from build123d import *

# Parameters (mm, degrees)
F0_R     = 38.1
F0_R_2   = 19.05
F1_DEPTH = 76.2
F2_R     = 9.52499
F4_R     = 31.75
F4_R_2   = 25.4
F5_DEPTH = 3.175
F6_R     = 3.17499
F8_R     = 19.05
F9_DEPTH = 152.4


# Not quite as in the source:
# - a fillet or chamfer is up to 0.001 mm smaller than in the source, because OpenCascade refuses the exact size


with BuildPart() as f1:
    # F0 (on Front) → F1 (new body, symmetric)
    with BuildSketch(Plane.XZ):
        Circle(F0_R)
        Circle(F0_R_2, mode=Mode.SUBTRACT)
    extrude(amount=F1_DEPTH, both=True)

    # F2 (radius 9.525 in the source; OpenCascade refuses exactly that, so slightly less here)
    f2_edges = [f1.edges().sort_by_distance(p)[0] for p in [
        (-38.1, -76.2, 0),
        (-19.05, -76.2, 0),
    ]]
    fillet(f2_edges, radius=F2_R)

    # F4 (on offset) → F5 (cut)
    with BuildSketch(Plane(origin=(0, 76.2, 0), x_dir=(-1, 0, 0), z_dir=(0, 1, 0))):
        Circle(F4_R)
        Circle(F4_R_2, mode=Mode.SUBTRACT)
    extrude(amount=-F5_DEPTH, mode=Mode.SUBTRACT)

    # F6 (radius 3.175 in the source; OpenCascade refuses exactly that, so slightly less here)
    f6_edges = [f1.edges().sort_by_distance(p)[0] for p in [
        (31.75, 73.025, 0),
        (25.4, 73.025, 0),
    ]]
    fillet(f6_edges, radius=F6_R)

    # F8 (on offset) → F9 (cut)
    with BuildSketch(Plane.YZ.offset(76.2)):
        Circle(F8_R)
    extrude(amount=-F9_DEPTH, mode=Mode.SUBTRACT)


solid = f1.part
Work out the finished part from the listing and answer in its coordinate system (mm). Give positions to 0.01 mm unless a question says otherwise; leave off trailing zeros. Loops run counter-clockwise (first coordinate to the right, second up) from the corner with the lowest first, then second, coordinate; pieces in that order, holes last. Notation, with made-up numbers: (-8, 13) -> (15, 13) arc R20 cw to (15, 36) -> close; hole circle Ø2 at (47, -17). An arc over 180 degrees is marked (long way). Use a Markdown table: item, result. Add a question column.
1. Determine the mould class of faces 1 (the cylindrical face through (10.241, -40.279, 16.063)), 2 (the cylindrical face through (-30.235, 3.762, -23.183)), 3 (the flat face through (-9, 76.2, 31)) for opening direction X: released by +X, released by -X, zero draft, split by the parting line, or undercut.
2. Section A-A on z = 0 is taken. State how many separate pieces and enclosed holes the cut face has, and give its area (3 significant figures).
3. Section B-B on y = -36 is taken. Determine the outline of the cut face in (x, z).
4. Flat-ended cylindrical pins translate along their axes: pin 1 Ø1 at (x, z) = (-28.5, -3.5) entering from +Y; pin 2 Ø6 at (x, z) = (23.5, -5.5) entering from -Y; pin 3 Ø1 at (x, y) = (11.5, 61) entering from +Z; pin 4 Ø17 at (x, z) = (5, -8.5) entering from +Y. Find the tip coordinate at first contact, or state that the pin passes through.
5. Find the intervals of material crossed by probe 1 along X at (y, z) = (60, 0); probe 2 along Z at (x, y) = (-8, -23), in increasing order.
Results below:
| question | item | result |
|---|---|---|
| 1 | face 1 | undercut |
| 1 | face 2 | split by the parting line |
| 1 | face 3 | zero draft |
| 2 | separate pieces | 4 |
| 2 | enclosed holes | 0 |
| 2 | area | 4,250 mm^2 |
| 3 | outline | circle Ø76.2 at (0, 0); hole circle Ø38.1 at (0, 0) |
| 4 | pin 1 | stops at y = 73.09 |
| 4 | pin 2 | stops at y = -76.09 |
| 4 | pin 3 | stops at z = 36.48 |
| 4 | pin 4 | passes through |
| 5 | probe 1 | x = -38.1 to -19.05, 19.05 to 38.1 |
| 5 | probe 2 | z = -37.25 to -17.29, 17.29 to 37.25 |
